```python
from build123d import *

# Parameters (mm, degrees)
SKIZZE1_W                       = 20
SKIZZE1_H                       = 11
AUFSATZ_LINEAR_AUSTRAGEN1_DEPTH = 11
SKIZZE2_R                       = 0.55
SCHNITT_LINEAR_AUSTRAGEN1_DEPTH = 0.5
AUFSATZ_LINEAR_AUSTRAGEN2_DEPTH = 0.2
LINEARES_MUSTER1_COUNT          = 2
LINEARES_MUSTER1_PITCH          = 10.16
LINEARES_MUSTER2_COUNT          = 2
LINEARES_MUSTER2_PITCH          = 17.78
LINEARES_MUSTER3_COUNT          = 2
LINEARES_MUSTER3_PITCH          = 7.62
LINEARES_MUSTER3_COPY_1_DEPTH   = 0.2
LINEARES_MUSTER3_COPY_2_DEPTH   = 0.2


with BuildPart() as part:
    # Skizze1 → Aufsatz-Linear austragen1 (new body)
    with BuildSketch(Plane.XY):
        with Locations((8.89, -3.8)):
            Rectangle(SKIZZE1_W, SKIZZE1_H)
    extrude(amount=AUFSATZ_LINEAR_AUSTRAGEN1_DEPTH)

    # Skizze2 → Schnitt-Linear austragen1 (cut)
    with BuildSketch(Plane.XY.offset(11)):
        Circle(SKIZZE2_R)
        with Locations((0, -7.62)):
            Circle(SKIZZE2_R)
    extrude(amount=-SCHNITT_LINEAR_AUSTRAGEN1_DEPTH, mode=Mode.SUBTRACT)

    # Skizze3 → Aufsatz-Linear austragen2 (add, symmetric)
    with BuildSketch(Plane(origin=(0, 0, 0), x_dir=(1, 0, 0), z_dir=(0, 1, 0))):
        Polygon((-0.45, 0), (-0.45, 3.05), (0, 3.5), (0.45, 3.05), (0.45, 0), align=None)
    aufsatz_linear_austragen2 = extrude(amount=AUFSATZ_LINEAR_AUSTRAGEN2_DEPTH, both=True)

    # Lineares Muster1: Aufsatz-Linear austragen2 ×2
    with Locations(*[(i * LINEARES_MUSTER1_PITCH, 0, 0) for i in range(1, LINEARES_MUSTER1_COUNT)]):
        add(aufsatz_linear_austragen2)

    # Lineares Muster2: Aufsatz-Linear austragen2 ×2
    with Locations(*[(i * LINEARES_MUSTER2_PITCH, 0, 0) for i in range(1, LINEARES_MUSTER2_COUNT)]):
        add(aufsatz_linear_austragen2)

    # Lineares Muster3: Aufsatz-Linear austragen2 ×2
    with Locations(*[(0, -i * LINEARES_MUSTER3_PITCH, 0) for i in range(1, LINEARES_MUSTER3_COUNT)]):
        add(aufsatz_linear_austragen2)

    # Lineares Muster3 copy 1 sketch → Lineares Muster3 copy 1 (add, symmetric)
    with BuildSketch(Plane(origin=(10.16, -7.62, 0), x_dir=(1, 0, 0), z_dir=(0, 1, 0))):
        Polygon((-0.45, 0), (-0.45, 3.05), (0, 3.5), (0.45, 3.05), (0.45, 0), align=None)
    extrude(amount=LINEARES_MUSTER3_COPY_1_DEPTH, both=True)

    # Lineares Muster3 copy 2 sketch → Lineares Muster3 copy 2 (add, symmetric)
    with BuildSketch(Plane(origin=(17.78, -7.62, 0), x_dir=(1, 0, 0), z_dir=(0, 1, 0))):
        Polygon((-0.45, 0), (-0.45, 3.05), (0, 3.5), (0.45, 3.05), (0.45, 0), align=None)
    extrude(amount=LINEARES_MUSTER3_COPY_2_DEPTH, both=True)


solid = part.part
```
Verification items for the finished model (mm, model axes). A direction names the side the tool comes from. Coordinates: 2 decimals unless noted, no trailing zeros. Loops run counter-clockwise (first coordinate to the right, second up) from the corner with the lowest first, then second, coordinate; pieces in that order, holes last. Notation, with made-up numbers: (6.25, 68) -> (29.25, 68) arc R22 cw to (29.25, 83) -> close; hole circle Ø5 at (-21, -33). An arc over 180 degrees is marked (long way). Put each result on its own line as item: value.
1. Thickness scan on line 1 (X direction, y = -7.75, z = -0.25); line 2 (Y direction, x = 0, z = 10.8); line 3 (Z direction, x = 9.25, y = 1). Record the ranges inside material, lowest first.
Result set:
line 1: x = -0.45 to 0.45, 9.71 to 10.61, 17.33 to 18.23
line 2: y = -9.3 to -8.17, -7.07 to -0.55, 0.55 to 1.7
line 3: z = 0 to 11
2. Section check A-A, the plane z = -1.5. Record the boundary of the cut face in (x, y).
Result set:
outline: (-0.45, -7.82) -> (0.45, -7.82) -> (0.45, -7.42) -> (-0.45, -7.42) -> close; (-0.45, -0.2) -> (0.45, -0.2) -> (0.45, 0.2) -> (-0.45, 0.2) -> close; (9.71, -7.82) -> (10.61, -7.82) -> (10.61, -7.42) -> (9.71, -7.42) -> close; (9.71, -0.2) -> (10.61, -0.2) -> (10.61, 0.2) -> (9.71, 0.2) -> close; (17.33, -7.82) -> (18.23, -7.82) -> (18.23, -7.42) -> (17.33, -7.42) -> close; (17.33, -0.2) -> (18.23, -0.2) -> (18.23, 0.2) -> (17.33, 0.2) -> close
3. Gauge pin test, flat ends, axial feed: P1, Ø5.5, axis at x = 13.5, y = -4, coming from the -Z side; P2, Ø1, axis at x = 17.5, z = -1, coming from the +Y side; P3, Ø1, axis at x = 10, z = -2.5, coming from the -Y side. Record the tip position at first contact, or that the pin passes through.
Result set:
P1: stops at z = 0
P2: stops at y = 0.2
P3: stops at y = -7.82
4. Mould release check, pull along Y, two halves, no side actions. Record for faces 1 (the face through (18, -7.42, -2)), 2 (the face through (10, -7.82, -2)), 3 (the face through (10, 0.2, -2)): pulls with the +Y half, pulls with the -Y half, needs draft (parallel to the pull), parting line crosses it, or undercut.
Result set:
face 1: undercut
face 2: pulls with the -Y half
face 3: pulls with the +Y half
5. Section check B-B, the plane y = -3.25. Record the boundary of the cut face in (x, z).
Result set:
outline: (-1.11, 0) -> (18.89, 0) -> (18.89, 11) -> (-1.11, 11) -> close
6. Tool access check on faces 4 (the face through (0, -0.2, -2)), 5 (the face through (0, 0.2, -2)), 6 (the face through (0, 0, 10.5)). Record the directions out of +Z, -Z, +X, -X, +Y, -Y that give a thin tool (end or side, any length) a straight path to the whole face; none if there is none.
Result set:
face 4: -Z, +X, -X
face 5: -Z, +X, -X, +Y
face 6: +Z
